The model under review builds one solid part; all positions refer to its coordinate system, in mm. Face numbers are marked on the shaded views. A direction names the side the tool comes from. Coordinates: 2 decimals unless noted, no trailing zeros. Loops run counter-clockwise (first coordinate to the right, second up) from the corner with the lowest first, then second, coordinate; pieces in that order, holes last. Notation, with made-up numbers: M 19,18.25 L 72,18.25 A19 cw 72,40.25 Z; hole C 59.5,83.5 d6. An arc over 180 degrees is marked long. Use one line per item in the form item = value.
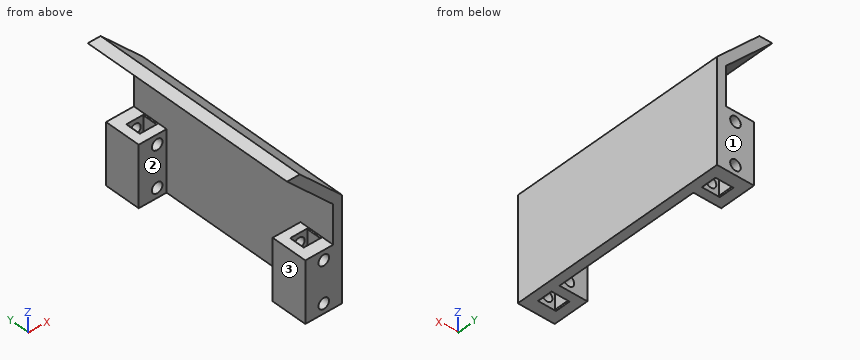
```python
from build123d import *

# Parameters (mm, degrees)
EXTRUDE_1_DEPTH     = 73.2
SKETCH_2_W          = 9.2
SKETCH_2_H          = 20
EXTRUDE_2_DEPTH     = 12
SKETCH_4_R          = 1.75
CUT_EXTRUDE_1_DEPTH = 20
SKETCH_7_W          = 5.45
SKETCH_7_H          = 6.4
SKETCH_7_W_2        = 5.35
CUT_EXTRUDE_2_DEPTH = 5
CHAMFER_1_SIZE      = 0.3


with BuildPart() as part:
    # 草图1 → 凸台-拉伸1 (new body)
    with BuildSketch(Plane(origin=(0, 0, 0), x_dir=(1, 0, 0), z_dir=(0, 1, 0))):
        Polygon((-12.5, -31), (1.5, -17), (1.5, 17), (-1.5, 17), (-1.5, -15.757359313), (-16.742640687, -31), align=None)
    extrude(amount=EXTRUDE_1_DEPTH)

    # 草图2 → 凸台-拉伸2 (add)
    with BuildSketch(Plane(origin=(0, 73.2, 0), x_dir=(1, 0, 0), z_dir=(0, 1, 0))):
        with Locations((-6.1, 7)):
            Rectangle(SKETCH_2_W, SKETCH_2_H)
    extrude_2 = extrude(amount=-EXTRUDE_2_DEPTH)

    # 草图4 → 切除-拉伸1 (cut)
    with BuildSketch(Plane(origin=(0, 73.2, 0), x_dir=(1, 0, 0), z_dir=(0, 1, 0))):
        with Locations(Location((-4.6, 13.8, 0), (0, 0, 270))):
            Circle(SKETCH_4_R)
        with Locations(Location((-4.6, 0.2, 0), (0, 0, 90))):
            Circle(SKETCH_4_R)
    cut_extrude_1 = extrude(amount=-CUT_EXTRUDE_1_DEPTH, mode=Mode.SUBTRACT)

    # 草图7 → 切除-拉伸2 (cut)
    with BuildSketch(Plane(origin=(0, 69.2, 0), x_dir=(1, 0, 0), z_dir=(0, 1, 0))):
        with Locations((-4.6, 0.2)):
            Rectangle(SKETCH_7_W, SKETCH_7_H)
        with Locations((-4.55, 13.8)):
            Rectangle(SKETCH_7_W_2, SKETCH_7_H)
    cut_extrude_2 = extrude(amount=-CUT_EXTRUDE_2_DEPTH, mode=Mode.SUBTRACT)

    # 镜向1: 凸台-拉伸2, 切除-拉伸1, 切除-拉伸2 across plane
    add(extrude_2.mirror(Plane.ZX.offset(36.6)))
    add(cut_extrude_1.mirror(Plane.ZX.offset(36.6)), mode=Mode.SUBTRACT)
    add(cut_extrude_2.mirror(Plane.ZX.offset(36.6)), mode=Mode.SUBTRACT)

    # 倒角1
    chamfer_1_edges = [part.edges().sort_by_distance(p)[0] for p in [
        (-7.325, 6.5, 3),
        (-1.875, 6.5, 3),
        (-7.225, 6.5, -17),
        (-1.875, 6.5, -17),
        (-7.325, 66.7, 3),
        (-1.875, 66.7, 3),
        (-7.225, 66.7, -17),
        (-1.875, 66.7, -17),
    ]]
    chamfer(chamfer_1_edges, length=CHAMFER_1_SIZE)


solid = part.part
```
1. Wall thickness on line 1 along X through (y, z) = (10, 0); line 2 along Z through (x, y) = (-4.6, 2.8); line 3 along X through (y, z) = (10, 7.5): over which ranges is each line inside the solid? List them lowest first. Write a range as from..to.
Response values:
line_1 = -10.7..-6.34, -2.86..1.5
line_2 = -17..-15.55, -12.05..-1.95, 1.55..3, 18.86..23.1
line_3 = -1.5..1.5
2. Add section C-C (x = 0.75). State the section outline as (y, z) points, then the cut area to 3 significant figures.
Response values:
outline = M 0,-17 L 73.2,-17 L 73.2,17.75 L 0,17.75 Z
area = 2,540 mm^2
3. Add section B-B (y = 50.5). State the section outline as (x, z) points, then the cut area to 3 significant figures.
Response values:
outline = M -16.74,31 L -1.5,15.76 L -1.5,-17 L 1.5,-17 L 1.5,17 L -12.5,31 Z
area = 162 mm^2
4. Insertion check: P1, Ø7.5, axis at x = -4.5, y = 68.5, coming from the +Z side; P2, Ø13, axis at y = 66, z = -9, coming from the -X side; P3, Ø4, axis at x = -3.5, y = 42.5, coming from the +Z side; P4, Ø3, axis at x = -4.6, z = -0.2, coming from the +Y side. Each pin has a flat end and moves straight along its axis. Give the tip position at first contact, or say it passes through.
Response values:
P1 = 26.75
P2 = -10.7
P3 = 24
P4 = through
5. Add section A-A (z = -0.2). Count the separate pieces of the cut face and the enclosed holes in it, then the cut area to 3 significant figures.
Response values:
separate_pieces = 3
enclosed_holes = 0
area = 337 mm^2
6. Machinability: for the marked faces 1, 2 and 3, which of the approach directions +Z, -Z, +X, -X, +Y, -Y give a long, thin tool a straight path to every point of the face, cutting with its end or side? Answer none if there is none.
Response values:
face_1 = +Z, -Z, +X, -X, +Y
face_2 = -Z, -X
face_3 = -Z, -X, +Y, -Y
